Verification items for the finished model (mm, model axes). Face numbers are marked on the shaded views. A direction names the side the tool comes from. Coordinates: 2 decimals unless noted, no trailing zeros. Order: outer loops, then holes, each group sorted by start corner. A loop starts at its lowest first (then second) coordinate and runs counter-clockwise, first axis right, second up.
Q1. Set-up check for the marked faces 5, 6 and 7: record each of +Z, -Z, +X, -X, +Y, -Y from which the full face is reachable in a straight line by a thin tool's end or side.
Q2. Draft check along X on the marked faces 1, 2, 3 and 4. Enter one of: pulls with the +X half, pulls with the -X half, needs draft (parallel to the pull), parting line crosses it, or undercut.
Q3. Thickness scan on line 1 (Y direction, x = -1, z = 5.75); line 2 (Y direction, x = 1.5, z = 2.25); line 3 (Y direction, x = 8.5, z = 4.75). Record the ranges inside material, lowest first.
Q4. Depth check by flat-ended pin: P1, Ø5.5, axis at y = -7.5, z = 2, coming from the +X side; P2, Ø1.5, axis at y = -7, z = 3.5, coming from the -X side; P3, Ø8.5, axis at x = -6, y = -7, coming from the +Z side; P4, Ø1, axis at x = -1.5, z = 7, coming from the +Y side. Enter the tip coordinate at first touch or a pass-through.
Q5. Cross-section at D-D, the plane x = -2.25. Record the boundary of the cut face in (y, z).
Q6. Cross-section at C-C, the plane y = 6. Record the boundary of the cut face in (x, z), and give its area (3 significant figures).
Q7. Cross-section at B-B, the plane z = 10.5. Record the boundary of the cut face in (x, y), and give its area (3 significant figures).
Q8. Cross-section at A-A, the plane z = 3.75. Record the boundary of the cut face in (x, y), and give its area (3 significant figures).
from build123d import *

# Parameters (mm, degrees)
F0_W     = 23
F0_H     = 9.5
F0_W_2   = 21
F0_H_2   = 7.5
F1_DEPTH = 2
F2_DEPTH = 5
F3_DEPTH = 7
F4_DEPTH = 2


with BuildPart() as f1:
    # F0 (on Top) → F1 (new body)
    with BuildSketch(Plane.XY):
        with BuildLine():
            Line((-0.8, 0.8), (-0.8, 11.4721401665))
            ThreePointArc((-0.8, 11.4721401665), (-8.1317279836, 8.1317279836), (-11.4721401665, 0.8))
            Line((-11.4721401665, 0.8), (-0.8, 0.8))
        make_face()
        with BuildLine():
            ThreePointArc((11.4721401665, 0.8), (8.1317279836, 8.1317279836), (0.8, 11.4721401665))
            Line((0.8, 11.4721401665), (0.8, 0.8))
            Line((0.8, 0.8), (11.4721401665, 0.8))
        make_face()
        with Locations((0, -27.25)):
            Rectangle(F0_W, F0_H)
        with Locations((0, -27.25)):
            Rectangle(F0_W_2, F0_H_2, mode=Mode.SUBTRACT)
        with BuildLine():
            Line((-0.8, -0.8), (-11.4721401665, -0.8))
            ThreePointArc((-11.4721401665, -0.8), (-8.1317279836, -8.1317279836), (-0.8, -11.4721401665))
            Line((-0.8, -11.4721401665), (-0.8, -0.8))
        make_face()
        with BuildLine():
            Line((0.8, -0.8), (0.8, -11.4721401665))
            ThreePointArc((0.8, -11.4721401665), (8.1317279836, -8.1317279836), (11.4721401665, -0.8))
            Line((11.4721401665, -0.8), (0.8, -0.8))
        make_face()
        with BuildLine():
            ThreePointArc((-0.8, -11.4721401665), (-8.1317279836, -8.1317279836), (-11.4721401665, -0.8))
            Line((-11.4721401665, -0.8), (-11.5, -0.8))
            Line((-11.5, -0.8), (-11.5, -22.5))
            Line((-11.5, -22.5), (11.5, -22.5))
            Line((11.5, -22.5), (11.5, -0.8))
            Line((11.5, -0.8), (11.4721401665, -0.8))
            ThreePointArc((11.4721401665, -0.8), (8.1317279836, -8.1317279836), (0.8, -11.4721401665))
            ThreePointArc((0.8, -11.4721401665), (0, -11.5), (-0.8, -11.4721401665))
        make_face()
        with BuildLine():
            ThreePointArc((0.8, 11.4721401665), (0, 11.5), (-0.8, 11.4721401665))
            Line((-0.8, 11.4721401665), (-0.8, 0.8))
            Line((-0.8, 0.8), (-11.4721401665, 0.8))
            ThreePointArc((-11.4721401665, 0.8), (-11.5, 0), (-11.4721401665, -0.8))
            Line((-11.4721401665, -0.8), (-0.8, -0.8))
            Line((-0.8, -0.8), (-0.8, -11.4721401665))
            ThreePointArc((-0.8, -11.4721401665), (0, -11.5), (0.8, -11.4721401665))
            Line((0.8, -11.4721401665), (0.8, -0.8))
            Line((0.8, -0.8), (11.4721401665, -0.8))
            ThreePointArc((11.4721401665, -0.8), (11.4930329312, -0.4002424797), (11.5, 0))
            ThreePointArc((11.5, 0), (11.4930329312, 0.4002424797), (11.4721401665, 0.8))
            Line((11.4721401665, 0.8), (0.8, 0.8))
            Line((0.8, 0.8), (0.8, 11.4721401665))
        make_face()
    extrude(amount=-F1_DEPTH)

    # F0 (on Top) → F2 (join)
    with BuildSketch(Plane.XY):
        with BuildLine():
            Line((-0.8, 0.8), (-0.8, 11.4721401665))
            ThreePointArc((-0.8, 11.4721401665), (-8.1317279836, 8.1317279836), (-11.4721401665, 0.8))
            Line((-11.4721401665, 0.8), (-0.8, 0.8))
        make_face()
        with BuildLine():
            ThreePointArc((11.4721401665, 0.8), (8.1317279836, 8.1317279836), (0.8, 11.4721401665))
            Line((0.8, 11.4721401665), (0.8, 0.8))
            Line((0.8, 0.8), (11.4721401665, 0.8))
        make_face()
        with BuildLine():
            Line((0.8, -0.8), (0.8, -11.4721401665))
            ThreePointArc((0.8, -11.4721401665), (8.1317279836, -8.1317279836), (11.4721401665, -0.8))
            Line((11.4721401665, -0.8), (0.8, -0.8))
        make_face()
        with BuildLine():
            Line((-0.8, -0.8), (-11.4721401665, -0.8))
            ThreePointArc((-11.4721401665, -0.8), (-8.1317279836, -8.1317279836), (-0.8, -11.4721401665))
            Line((-0.8, -11.4721401665), (-0.8, -0.8))
        make_face()
        with Locations((0, -27.25)):
            Rectangle(F0_W, F0_H)
        with Locations((0, -27.25)):
            Rectangle(F0_W_2, F0_H_2, mode=Mode.SUBTRACT)
    extrude(amount=F2_DEPTH)

    # F3 (add): a face of the model
    f3_faces = [f1.faces().sort_by_distance(p)[0] for p in [
        (0, -22.7488473428, 5),
    ]]
    extrude(f3_faces, amount=F3_DEPTH)

    # F0 (on Top) → F4 (join)
    with BuildSketch(Plane.XY):
        with Locations((0, -27.25)):
            Rectangle(F0_W_2, F0_H_2)
    extrude(amount=-F4_DEPTH)


solid = f1.part
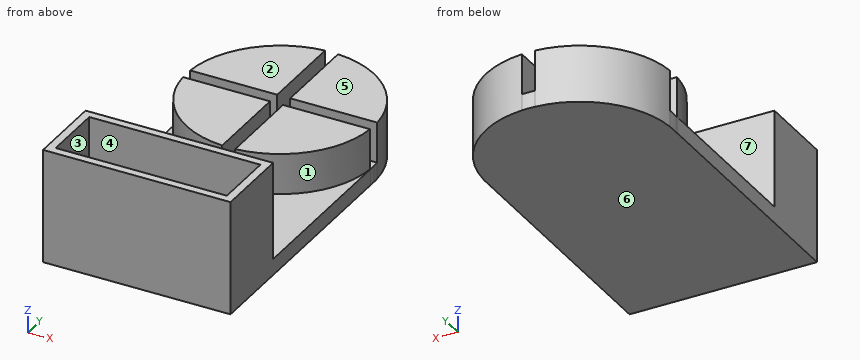
Check values:
1. face 5: +Z, +X, -X, +Y
1. face 6: -Z, +X, -X, +Y, -Y
1. face 7: +Z, +X, -X
2. face 1: pulls with the +X half
2. face 2: needs draft
2. face 3: undercut
2. face 4: undercut
3. line 1: y = -32 to -31, -23.5 to -22.5
3. line 2: y = -32 to -31, -23.5 to -22.5, -11.4 to -0.8, 0.8 to 11.4
3. line 3: y = -32 to -31, -23.5 to -22.5, -7.75 to -0.8, 0.8 to 7.75
4. P1: stops at x = 11.5
4. P2: stops at x = -9.65
4. P3: stops at z = 5
4. P4: stops at y = -22.5
5. outline: (-32, -2) - (11.28, -2) - (11.28, 5) - (0.8, 5) - (0.8, 0) - (-0.8, 0) - (-0.8, 5) - (-11.28, 5) - (-11.28, 0) - (-22.5, 0) - (-22.5, 12) - (-23.5, 12) - (-23.5, 0) - (-31, 0) - (-31, 12) - (-32, 12) - close
6. outline: (-9.81, -2) - (9.81, -2) - (9.81, 5) - (0.8, 5) - (0.8, 0) - (-0.8, 0) - (-0.8, 5) - (-9.81, 5) - close
6. area: 129 mm2
7. outline: (-11.5, -32) - (11.5, -32) - (11.5, -22.5) - (-11.5, -22.5) - close; hole (-10.5, -31) - (10.5, -31) - (10.5, -23.5) - (-10.5, -23.5) - close
7. area: 61.0 mm2
8. outline: (-11.5, -32) - (11.5, -32) - (11.5, -22.5) - (-11.5, -22.5) - close; (-11.47, -0.8) arc R11.5 ccw to (-0.8, -11.47) - (-0.8, -0.8) - close; (-11.47, 0.8) - (-0.8, 0.8) - (-0.8, 11.47) arc R11.5 ccw to start; (0.8, -11.47) arc R11.5 ccw to (11.47, -0.8) - (0.8, -0.8) - close; (0.8, 0.8) - (11.47, 0.8) arc R11.5 ccw to (0.8, 11.47) - close; hole (-10.5, -31) - (10.5, -31) - (10.5, -23.5) - (-10.5, -23.5) - close
8. area: 405 mm2
